from build123d import *
from OCP.BRepFilletAPI import BRepFilletAPI_MakeChamfer

# Parameters (mm, degrees)
SKETCH2_R          = 8.5725
EXTRUDE1_DEPTH     = 10.414
EXTRUDE1_DRAFT     = 1.5
CHAMFER1_SIZE      = 0.705555556
CHAMFER1_SIZE2     = 0.724776351
CHAMFER1_SIZE2_2   = 0.687787076
SKETCH6_W          = 11.938
SKETCH6_H          = 11.938
EXTRUDE2_DEPTH     = 10.922
CUT_EXTRUDE1_DEPTH = 10.922


with BuildPart() as part:
    # Sketch2 → Extrude1 (with draft: the straight prism first)
    with BuildSketch(Plane(origin=(10.668, 0, 0), x_dir=(0, 0, -1), z_dir=(1, 0, 0))):
        Circle(SKETCH2_R)
    extrude(amount=-EXTRUDE1_DEPTH)
    # Extrude1: the draft: its side faces are tilted about the plane it starts from
    extrude1_sides = [part.faces().sort_by_distance(p)[0] for p in [
        (5.461, 0, 8.5725),
    ]]
    draft(extrude1_sides, Plane(origin=(10.668, 0, 0), x_dir=(0, 0, -1), z_dir=(1, 0, 0)), EXTRUDE1_DRAFT)

    # Chamfer1: one chamfer whose edges measure the first distance from different faces: ONE call of the kernel's chamfer builder (chamfer() names one face for all edges)
    chamfer1_edges_1 = [part.edges().sort_by_distance(p)[0] for p in [
        (10.668, 0, 8.5725),
    ]]
    chamfer1_side_1 = [part.faces().sort_by_distance(p)[0] for p in [
        (5.461, 0, 8.708850094),
    ]]
    chamfer1_edges_2 = [part.edges().sort_by_distance(p)[0] for p in [
        (0.254, 0, 8.845200187),
    ]]
    chamfer1_side_2 = [part.faces().sort_by_distance(p)[0] for p in [
        (0.254, 0, 0),
    ]]
    chamfer1 = BRepFilletAPI_MakeChamfer(part.part.solid().wrapped)
    for e in chamfer1_edges_1:
        chamfer1.Add(CHAMFER1_SIZE, CHAMFER1_SIZE2, e.wrapped, chamfer1_side_1[0].wrapped)  # the first distance lies on this face
    for e in chamfer1_edges_2:
        chamfer1.Add(CHAMFER1_SIZE, CHAMFER1_SIZE2_2, e.wrapped, chamfer1_side_2[0].wrapped)  # the first distance lies on this face
    add(Compound.cast(chamfer1.Shape()), mode=Mode.REPLACE)

    # Sketch6 → Extrude2 (add)
    with BuildSketch(Plane.ZY.offset(-0.254)):
        Rectangle(SKETCH6_W, SKETCH6_H)
    extrude(amount=EXTRUDE2_DEPTH)

    # Sketch7 → Cut-Extrude1 (cut)
    with BuildSketch(Plane.ZY.offset(10.668)):
        Polygon((4.47675, 5.969), (5.969, 4.47675), (5.969, 5.969), align=None)
        Polygon((5.969, -4.47675), (4.47675, -5.969), (5.969, -5.969), align=None)
        Polygon((-5.969, -4.47675), (-4.47675, -5.969), (-5.969, -5.969), align=None)
        Polygon((-5.969, 4.47675), (-4.47675, 5.969), (-5.969, 5.969), align=None)
    extrude(amount=-CUT_EXTRUDE1_DEPTH, mode=Mode.SUBTRACT)


solid = part.part
Can you work these out from the model? Positions are in its coordinate system, mm. A direction names the side the tool comes from. Give positions to 0.01 mm unless a question says otherwise; leave off trailing zeros. Loops run counter-clockwise (first coordinate to the right, second up) from the corner with the lowest first, then second, coordinate; pieces in that order, holes last. Notation, with made-up numbers: (-12.5, 79) -> (23.5, 79) arc R21 cw to (23.5, 110) -> close; hole circle Ø10 at (-4, -17.5). An arc over 180 degrees is marked (long way). Use one line per item in the form item = value.
1) If we section it at B-B (x = -8.5): Please give me the cut outline in (y, z), plus the area to 3 significant figures.
Answers:
outline = (-5.97, -4.48) -> (-4.48, -5.97) -> (4.48, -5.97) -> (5.97, -4.48) -> (5.97, 4.48) -> (4.48, 5.97) -> (-4.48, 5.97) -> (-5.97, 4.48) -> close
area = 138 mm²
2) Will these pins go through, and if not, where does the flat tip stop? pin 1 (6 mm diameter, centred on x = -6.5, y = 1.5, fed in from +Z); pin 2 (10 mm diameter, centred on x = -7, z = 0.5, fed in from +Y); pin 3 (1 mm diameter, centred on x = 5.5, z = -5.5, fed in from -Y).
Answers:
pin_1 = 5.97
pin_2 = 5.97
pin_3 = -7.13
3) I need wall thicknesses on line 1 along X through (y, z) = (2.5, -7); line 2 along Z through (x, y) = (-1, -3.25). Which ranges of each line are inside material? Lowest first, please.
Answers:
line_1 = 0.25 to 10.67
line_2 = -5.97 to 5.97
4) If we section it at D-D (x = 8.5): Please give me the cut outline in (y, z).
Answers:
outline = circle Ø17.26 at (0, 0)
5) For faces 1 (the face through (-5.283, -5.212, 5.233)), 2 (the face through (-5.283, -5.212, -5.233)), 3 (the face through (-5, -5.969, 0)), 4 (the face through (-5, 5.969, 0)), which set-ups out of +Z, -Z, +X, -X, +Y, -Y let a thin tool reach every point of the face, with its end or its side?
Answers:
face_1 = +Z, -X, -Y
face_2 = -Z, -X, -Y
face_3 = +Z, -Z, -X, -Y
face_4 = +Z, -Z, -X, +Y
6) If we section it at A-A (y = 0): Please give me the cut outline in (x, z), plus the area to 3 significant figures.
Answers:
outline = (-10.67, -5.97) -> (0.25, -5.97) -> (0.25, -8.14) -> (0.94, -8.83) -> (9.96, -8.59) -> (10.67, -7.85) -> (10.67, 7.85) -> (9.96, 8.59) -> (0.94, 8.83) -> (0.25, 8.14) -> (0.25, 5.97) -> (-10.67, 5.97) -> close
area = 311 mm²
